```python
from build123d import *

# Parameters (mm, degrees)
SKETCH_1_R                  = 10
EXTRUDE_1_DEPTH             = 21
SKETCH_2_R                  = 6.5
CUT_EXTRUDE_1_DEPTH         = 15
M4X0_71_D                   = 3.3
M4X0_71_DEPTH               = 5
M4X0_71_TIP                 = 0.991420021
M3X0_51_D                   = 2.5
M3X0_51_DEPTH               = 6
HOLE_WIZARD_M31_D           = 3.4
HOLE_WIZARD_M31_CBORE_D     = 6.7
HOLE_WIZARD_M31_CBORE_DEPTH = 1.8


with BuildPart() as part:
    # Эскиз1 → Бобышка-Вытянуть1 (new body)
    with BuildSketch(Plane.XY):
        with Locations(Location((0, 0, 0), (0, 0, 180))):
            Circle(SKETCH_1_R)
    extrude(amount=EXTRUDE_1_DEPTH)

    # Эскиз2 → Вырез-Вытянуть1 (cut)
    with BuildSketch(Plane.XY.offset(21)):
        Circle(SKETCH_2_R)
    extrude(amount=-CUT_EXTRUDE_1_DEPTH, mode=Mode.SUBTRACT)

    # Отверстие обработанное метчиком M4x0.71
    with Locations(Plane(origin=(-10, 0, 0), x_dir=(0, 0, -1), z_dir=(-1, 0, 0))):
        with Locations((-14, 0)):
            Hole(M4X0_71_D / 2, depth=M4X0_71_DEPTH)
            with Locations((0, 0, -(M4X0_71_DEPTH + M4X0_71_TIP / 2))):  # 118° drill point
                Cone(0, M4X0_71_D / 2, M4X0_71_TIP, mode=Mode.SUBTRACT)

    # Отверстие обработанное метчиком M3x0.51
    with Locations(Plane(origin=(0, 0, 0), x_dir=(-1, 0, 0), z_dir=(0, 0, -1))):
        with Locations((-4.242640687, 4.242640687), (4.242640687, 4.242640687), (4.242640687, -4.242640687), (-4.242640687, -4.242640687)):
            Hole(M3X0_51_D / 2, depth=M3X0_51_DEPTH)

    # Цековка для  винта с полукруглой головкой M31 (through all)
    with Locations(Plane(origin=(0, 0, 0), x_dir=(-1, 0, 0), z_dir=(0, 0, -1))):
        with Locations((0, 0)):
            CounterBoreHole(HOLE_WIZARD_M31_D / 2, HOLE_WIZARD_M31_CBORE_D / 2, HOLE_WIZARD_M31_CBORE_DEPTH)


solid = part.part
```
Model file for the job. Use its own axes, mm. A direction names the side the tool comes from. Give positions to 0.01 mm unless a question says otherwise; leave off trailing zeros. Loops run counter-clockwise (first coordinate to the right, second up) from the corner with the lowest first, then second, coordinate; pieces in that order, holes last. Notation, with made-up numbers: (-6, -33) -> (7, -33) arc R14 ccw to (7, -21) -> close; hole circle Ø2 at (87.25, -29.5). An arc over 180 degrees is marked (long way). Write each question's results on one line, items separated by ' | '.
(1) Tool access for faces 1 (the cylindrical face through (6, -2.5, 13.6)), 2 (the cylindrical face through (-8.12, -0.07, 12.35)), 3 (the flat face through (-5, 5, 6)): list every direction of +Z, -Z, +X, -X, +Y, -Y with a clear straight run to the whole face (end or side of a thin tool).
Geometry results:
face 1: +Z | face 2: -X | face 3: -Z
(2) Pull direction Y, two halves, no side cores. Call faces 4 (the flat face through (-7, 0, 21)), 5 (the flat face through (1.4, -1.4, 6)), 6 (the cylindrical face through (10, 0, 10)), 7 (the cylindrical face through (-5.235, 3.482, 3.042)): released by +Y, released by -Y, zero draft, split by the parting line, or undercut.
Geometry results:
face 4: zero draft | face 5: undercut | face 6: split by the parting line | face 7: undercut
(3) Flat gauge pins, fed straight in: pin 1 Ø1.5 at (y, z) = (5, 17.5) entering from -X; pin 2 Ø4 at (y, z) = (3, 13.5) entering from +X; pin 3 Ø4 at (y, z) = (-4.5, 19) entering from -X. Where does each tip first touch, or does it go through?
Geometry results:
pin 1: stops at x = -9.05 | pin 2: stops at x = 9.95 | pin 3: stops at x = -9.68
(4) Cut at D-D on x = -2.25. List the corners of the cut face in (y, z).
Geometry results:
outline: (-9.74, 0) -> (-2.48, 0) -> (-2.48, 1.8) -> (2.48, 1.8) -> (2.48, 0) -> (9.74, 0) -> (9.74, 21) -> (6.1, 21) -> (6.1, 6) -> (-6.1, 6) -> (-6.1, 21) -> (-9.74, 21) -> close
(5) Cut at C-C on z = 7.25. List the corners of the cut face in (x, y), and give its area (3 significant figures).
Geometry results:
outline: circle Ø20 at (0, 0); hole circle Ø13 at (0, 0) | area: 181 mm²
(6) Cut at A-A on x = 0. List the corners of the cut face in (y, z), and give its area (3 significant figures).
Geometry results:
outline: (-10, 0) -> (-3.35, 0) -> (-3.35, 1.8) -> (-1.7, 1.8) -> (-1.7, 6) -> (-6.5, 6) -> (-6.5, 21) -> (-10, 21) -> close; (1.7, 1.8) -> (3.35, 1.8) -> (3.35, 0) -> (10, 0) -> (10, 21) -> (6.5, 21) -> (6.5, 6) -> (1.7, 6) -> close | area: 199 mm²
(7) Cut at B-B on y = 0. List the corners of the cut face in (x, z).
Geometry results:
outline: (-10, 0) -> (-3.35, 0) -> (-3.35, 1.8) -> (-1.7, 1.8) -> (-1.7, 6) -> (-6.5, 6) -> (-6.5, 12.35) -> (-10, 12.35) -> close; (-10, 15.65) -> (-6.5, 15.65) -> (-6.5, 21) -> (-10, 21) -> close; (1.7, 1.8) -> (3.35, 1.8) -> (3.35, 0) -> (10, 0) -> (10, 21) -> (6.5, 21) -> (6.5, 6) -> (1.7, 6) -> close
(8) Probe line 1 along Y through (x, z) = (0, 3.1); line 2 along Y through (x, z) = (-3.75, 2.5); line 3 along Z through (x, y) = (0.25, 2.75). List the from-to ranges inside material, lowest first.
Geometry results:
line 1: y = -10 to -1.7, 1.7 to 10 | line 2: y = -9.27 to -5.39, -3.09 to 3.09, 5.39 to 9.27 | line 3: z = 1.8 to 6
